Design review of the part built by this model. Coordinates are the model's own, in mm. Coordinates: 2 decimals unless noted, no trailing zeros. Loops run counter-clockwise (first coordinate to the right, second up) from the corner with the lowest first, then second, coordinate; pieces in that order, holes last.
Q1. Add section D-D on x = 6. Give the boundary of the cut face in (y, z), and give its area (3 significant figures).
Q2. Add section B-B on z = -25.1. Give the boundary of the cut face in (x, y).
Q3. Wall thickness on probe 1 along X at (y, z) = (0.2, 23.4); probe 2 along X at (y, z) = (0.3, -24.5); probe 3 along Z at (x, y) = (12.5, 0.65): over which ranges is each line inside the solid? List them lowest first.
Q4. Draft analysis for pull direction Z (two halves, no side actions). For faces 1 (the face through (0, 0, 0)), 2 (the face through (13.57, 0.35, -25.6)), 3 (the face through (-12.083, 0.355, 24.324)), state which applies: released by +Z, released by -Z, zero draft, split by the parting line, or undercut.
Q5. Add section C-C on z = 23.4. Give the boundary of the cut face in (x, y), and give its area (3 significant figures).
Q6. For P1, Ø1.6, axis at x = -11.7, z = 23.4, coming from the -Y side, flat-tipped, find the tip position at first contact; note if it passes through.
Q7. Add section A-A on y = 0.35. Give the boundary of the cut face in (x, z).
```python
from build123d import *

# Parameters (mm, degrees)
SKETCH2_W          = 30
SKETCH2_H          = 54.2
CIRCUITBOARD_DEPTH = 0.7
SKETCH3_W          = 3.3
SKETCH3_H          = 10.5
SKETCH3_W_2        = 6.4
SKETCH3_H_2        = 2.5
CUT_EXTRUDE1_DEPTH = 31.982252985
FILLET2_R          = 5
SKETCH4_R          = 1
SCREWHOLES_DEPTH   = 31.982252985


with BuildPart() as part:
    # Sketch2 → CircuitBoard (new body)
    with BuildSketch(Plane(origin=(0, 0, 0), x_dir=(1, 0, 0), z_dir=(0, 1, 0))):
        Rectangle(SKETCH2_W, SKETCH2_H)
    extrude(amount=CIRCUITBOARD_DEPTH)

    # Sketch3 → Cut-Extrude1 (cut, through all)
    with BuildSketch(Plane(origin=(0, 0.7, 0), x_dir=(1, 0, 0), z_dir=(0, 1, 0))):
        with Locations((-13.35, 11.85)):
            Rectangle(SKETCH3_W, SKETCH3_H)
        with Locations((-7.1, -25.85)):
            Rectangle(SKETCH3_W_2, SKETCH3_H_2)
    cut_extrude1 = extrude(amount=-CUT_EXTRUDE1_DEPTH, mode=Mode.SUBTRACT)

    # Cut_Mirror: Cut-Extrude1 across plane
    add(cut_extrude1.mirror(Plane(origin=(0, 0, 0), x_dir=(0, 0, 1), z_dir=(1, 0, 0))), mode=Mode.SUBTRACT)

    # Cut_Mirror at the second plane: Cut-Extrude1 across plane
    add(cut_extrude1.mirror(Plane.ZX), mode=Mode.SUBTRACT)

    # Fillet2
    # the kernel refuses this fillet: 5 mm, written as the material it takes off along each edge
    with BuildSketch(Plane(origin=(-15, -12.477479713, 27.1), x_dir=(0, 0, -1), z_dir=(0, 1, 0))) as fillet2_piece_1:
        with BuildLine():
            CenterArc((4.990991885, -5), FILLET2_R, 90, 86.560187232)
            Line((0, -4.7), (-0.099819838, -4.694))
            ThreePointArc((-0.099819838, -4.694), (-0.1, -2.35), (-0.1, 0))
            Line((-0.1, 0), (0, 0.1))
            Line((0, 0.1), (4.990991885, 0.1))
            Line((4.990991885, 0.1), (4.990991885, 0))
        make_face()
    extrude(amount=25.654959427, mode=Mode.SUBTRACT)
    with BuildSketch(Plane(origin=(15, -12.477479713, 27.1), x_dir=(-1, 0, 0), z_dir=(0, 1, 0))) as fillet2_piece_2:
        with BuildLine():
            CenterArc((5, -4.990991885), FILLET2_R, 93.439812768, 86.560187232)
            Line((0, -4.990991885), (-0.1, -4.990991885))
            Line((-0.1, -4.990991885), (-0.1, 0))
            Line((-0.1, 0), (0, 0.1))
            ThreePointArc((0, 0.1), (2.35, 0.1), (4.694, 0.099819838))
            Line((4.694, 0.099819838), (4.7, 0))
        make_face()
    extrude(amount=25.654959427, mode=Mode.SUBTRACT)
    with BuildSketch(Plane(origin=(15, -12.5, -27.1), x_dir=(-1, 0, 0), z_dir=(0, 1, 0))) as fillet2_piece_3:
        with BuildLine():
            CenterArc((FILLET2_R, FILLET2_R), FILLET2_R, 180, 90)
            Line((0, FILLET2_R), (-FILLET2_R * 0.02, FILLET2_R))
            Line((-FILLET2_R * 0.02, FILLET2_R), (-FILLET2_R * 0.02, -FILLET2_R * 0.02))
            Line((-FILLET2_R * 0.02, -FILLET2_R * 0.02), (FILLET2_R, -FILLET2_R * 0.02))
            Line((FILLET2_R, -FILLET2_R * 0.02), (FILLET2_R, 0))
        make_face()
    extrude(amount=25.7, mode=Mode.SUBTRACT)
    with BuildSketch(Plane(origin=(-15, -12.5, -27.1), x_dir=(1, 0, 0), z_dir=(0, 1, 0))) as fillet2_piece_4:
        with BuildLine():
            CenterArc((FILLET2_R, -FILLET2_R), FILLET2_R, 90, 90)
            Line((0, -FILLET2_R), (-FILLET2_R * 0.02, -FILLET2_R))
            Line((-FILLET2_R * 0.02, -FILLET2_R), (-FILLET2_R * 0.02, FILLET2_R * 0.02))
            Line((-FILLET2_R * 0.02, FILLET2_R * 0.02), (FILLET2_R, FILLET2_R * 0.02))
            Line((FILLET2_R, FILLET2_R * 0.02), (FILLET2_R, 0))
        make_face()
    extrude(amount=25.7, mode=Mode.SUBTRACT)

    # Sketch4 → ScrewHoles (cut, through all)
    with BuildSketch(Plane(origin=(0, 0.7, 0), x_dir=(1, 0, 0), z_dir=(0, 1, 0))):
        with Locations(Location((-11.7, 25.1, 0), (0, 0, 270))):
            Circle(SKETCH4_R)
        with Locations(Location((-11.7, -23.4, 0), (0, 0, 270))):
            Circle(SKETCH4_R)
    screwholes = extrude(amount=-SCREWHOLES_DEPTH, mode=Mode.SUBTRACT)

    # ScrewHoles_Mirror: ScrewHoles across plane
    add(screwholes.mirror(Plane(origin=(0, 0, 0), x_dir=(0, 0, 1), z_dir=(1, 0, 0))), mode=Mode.SUBTRACT)

    # ScrewHoles_Mirror at the second plane: ScrewHoles across plane
    add(screwholes.mirror(Plane.ZX), mode=Mode.SUBTRACT)


solid = part.part
```
Entries:
1. outline: (0, -27.1) - (0.7, -27.1) - (0.7, 24.6) - (0, 24.6) - close
1. area: 36.2 mm2
2. outline: (-14, 0) - (-12.7, 0) - (-12.7, 0.7) - (-14, 0.7) - close; (-10.7, 0) - (10.7, 0) - (10.7, 0.7) - (-10.7, 0.7) - close; (12.7, 0) - (14, 0) - (14, 0.7) - (12.7, 0.7) - close
3. probe 1: x = -14.83 to -12.7, -10.7 to 10.7, 12.7 to 14.83
3. probe 2: x = -14.39 to -12.5, -10.9 to 10.9, 12.5 to 14.39
3. probe 3: z = -26.43 to -25.7, -24.5 to -17.1, -6.6 to 22.8, 24 to 26.44
4. face 1: zero draft
4. face 2: released by -Z
4. face 3: undercut
5. outline: (-14.83, 0) - (-12.7, 0) - (-12.7, 0.7) - (-14.83, 0.7) - close; (-10.7, 0) - (10.7, 0) - (10.7, 0.7) - (-10.7, 0.7) - close; (12.7, 0) - (14.83, 0) - (14.83, 0.7) - (12.7, 0.7) - close
5. area: 18.0 mm2
6. P1: passes through
7. outline: (-15, -22.1) arc R5 ccw to (-10, -27.1) - (10, -27.1) arc R5 ccw to (15, -22.1) - (15, -17.1) - (11.7, -17.1) - (11.7, -6.6) - (15, -6.6) - (15, 22.11) arc R5 ccw to (10.3, 27.1) - (10.3, 24.6) - (3.9, 24.6) - (3.9, 27.1) - (-3.9, 27.1) - (-3.9, 24.6) - (-10.3, 24.6) - (-10.3, 27.1) arc R5 ccw to (-15, 22.11) - (-15, -6.6) - (-11.7, -6.6) - (-11.7, -17.1) - (-15, -17.1) - close; hole circle Ø2 at (-11.7, -25.1); hole circle Ø2 at (-11.7, 23.4); hole circle Ø2 at (11.7, -25.1); hole circle Ø2 at (11.7, 23.4)
